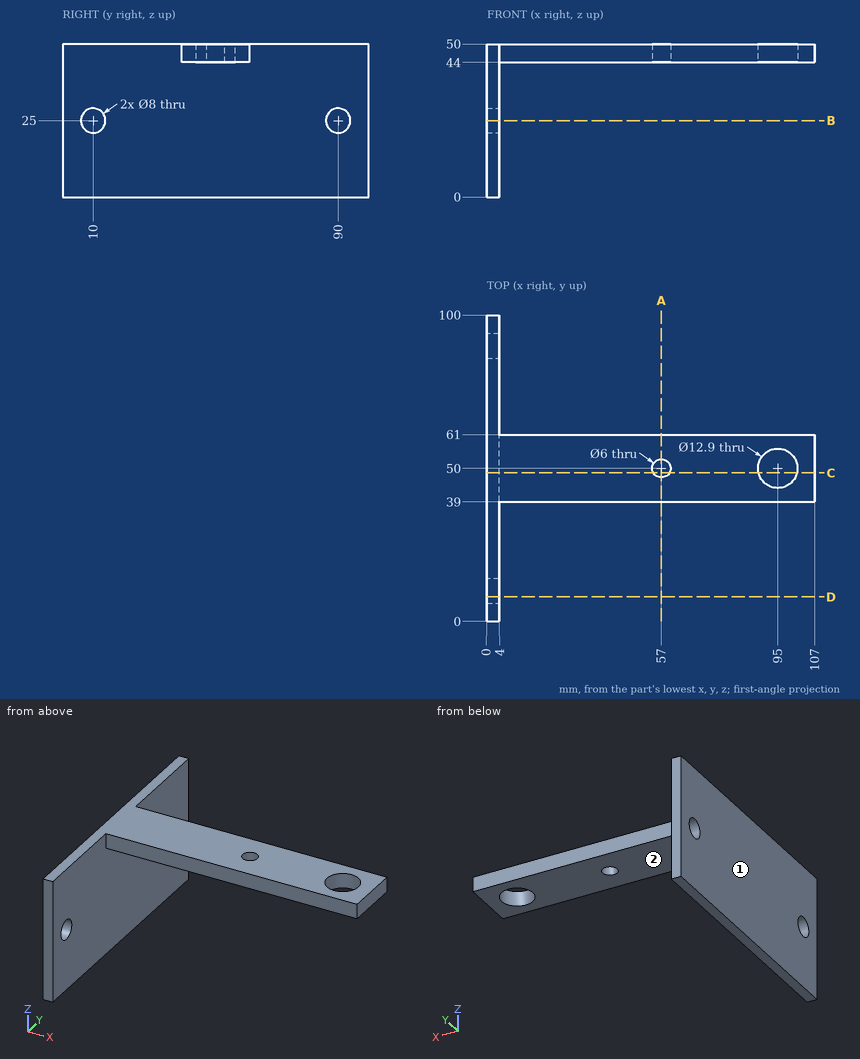
Job drawing, mm, ordinate dimensions from the low corner. One solid piece. A direction names the side the tool comes from. Coordinates: 2 decimals unless noted, no trailing zeros. Write each loop counter-clockwise with the first axis right and the second up, starting at its lowest first coordinate (ties: lowest second). Pieces come first, ordered by that corner, then holes. Notation, with made-up numbers: (-30.5, 60) -> (24.5, 60) arc R19 ccw to (24.5, 82) -> close; hole circle Ø9 at (80.25, 2). An arc over 180 degrees is marked (long way). Use CSV: the item, a comma, the result in double quotes. Start each with the question number.
Item 1: Drop flat-ended pins along their axis: P1, Ø4, axis at x = 15, z = 43.5, coming from the -Y side; P2, Ø6.5, axis at x = 41.5, y = 46.5, coming from the -Z side; P3, Ø13, axis at y = 10, z = 25, coming from the +X side. Give the stop position or say it passes through.
Item 2: Band-saw the part on B-B, the plane z = 25. Write the cut outline in (x, y), plus the area to 3 significant figures.
Item 3: Band-saw the part on D-D, the plane y = 8. Write the cut outline in (x, z), plus the area to 3 significant figures.
Item 4: Band-saw the part on C-C, the plane y = 48.5. Write the cut outline in (x, z), plus the area to 3 significant figures.
Item 5: Tool access for the marked faces 1 and 2: list every direction of +Z, -Z, +X, -X, +Y, -Y with a clear straight run to the whole face (end or side of a thin tool).
Item 6: Band-saw the part on A-A, the plane x = 57. Write the cut outline in (y, z), plus the area to 3 significant figures.
Item 7: Wall check: probe 1 along X at (y, z) = (50, 47.1); probe 2 along X at (y, z) = (56.5, 29.5); probe 3 along Y at (x, z) = (38, 44.5). Give the ranges that are in metal, low to high.
Response values:
1,P1,"stops at y = 39"
1,P2,"stops at z = 44"
1,P3,"stops at x = 4"
2,outline,"(0, 0) -> (4, 0) -> (4, 6) -> (0, 6) -> close; (0, 14) -> (4, 14) -> (4, 86) -> (0, 86) -> close; (0, 94) -> (4, 94) -> (4, 100) -> (0, 100) -> close"
2,area,"336 mm2"
3,outline,"(0, 0) -> (4, 0) -> (4, 21.54) -> (0, 21.54) -> close; (0, 28.46) -> (4, 28.46) -> (4, 50) -> (0, 50) -> close"
3,area,"172 mm2"
4,outline,"(0, 0) -> (4, 0) -> (4, 44) -> (54.4, 44) -> (54.4, 50) -> (0, 50) -> close; (59.6, 44) -> (88.73, 44) -> (88.73, 50) -> (59.6, 50) -> close; (101.27, 44) -> (107, 44) -> (107, 50) -> (101.27, 50) -> close"
4,area,"712 mm2"
5,face 1,"+Z, -Z, -X, +Y, -Y"
5,face 2,"-Z, +X, +Y, -Y"
6,outline,"(39, 44) -> (47, 44) -> (47, 50) -> (39, 50) -> close; (53, 44) -> (61, 44) -> (61, 50) -> (53, 50) -> close"
6,area,"96.0 mm2"
7,probe 1,"x = 0 to 54, 60 to 88.55, 101.45 to 107"
7,probe 2,"x = 0 to 4"
7,probe 3,"y = 39 to 61"
